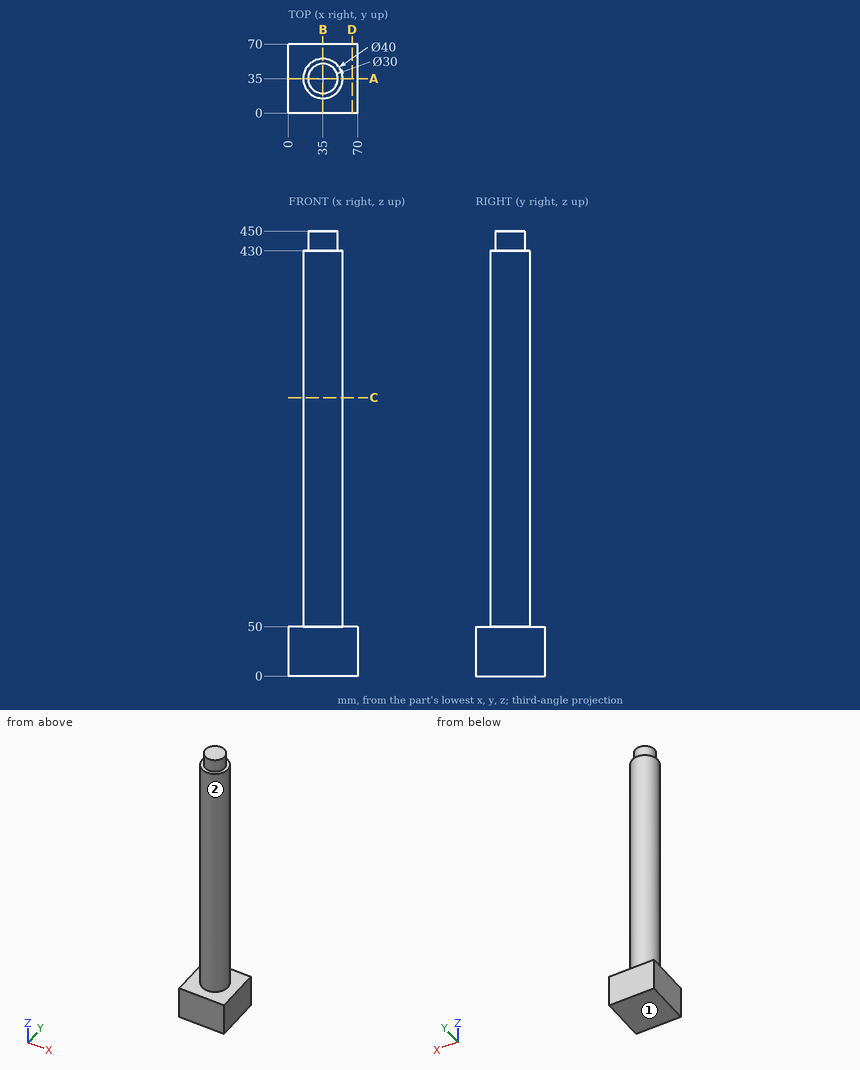
The figure shows three views and two pictorial views of one solid part (mm, origin at its lowest corner). Answer the questions. A direction names the side the tool comes from. Coordinates: 2 decimals unless noted, no trailing zeros. Write each loop counter-clockwise with the first axis right and the second up, starting at its lowest first coordinate (ties: lowest second). Pieces come first, ordered by that corner, then holes. Notation, with made-up numbers: (9, 13.25) -> (33, 13.25) arc R29 ccw to (33, 51.25) -> close; hole circle Ø5 at (-7, -14). An arc over 180 degrees is marked (long way). Answer as a JSON object with one key per item and string values.
Q1. Consider line 1 (Z direction, x = 47, y = 15); line 2 (Z direction, x = 47.5, y = 45); line 3 (Y direction, x = 47, z = 386.5). Determine where each line is inside the solid, lowest interval first. Write a range as [from, to].
The answers:
{"line 1": "z = [0, 50]", "line 2": "z = [0, 430]", "line 3": "y = [19, 51]"}
Q2. The part is cut by section C-C on z = 281.5. Give the vertices of the cut face in (x, y).
The answers:
{"outline": "circle Ø40 at (35, 35)"}
Q3. Flat-ended cylindrical pins translate along their axes: pin 1 Ø2 at (y, z) = (21, 121.5) entering from +X; pin 2 Ø2 at (x, z) = (36.5, 273.5) entering from +Y; pin 3 Ø3 at (x, y) = (54.5, 8.5) entering from +Z. Find the tip coordinate at first contact, or state that the pin passes through.
The answers:
{"pin 1": "stops at x = 50.2", "pin 2": "stops at y = 54.99", "pin 3": "stops at z = 50"}
Q4. The part is cut by section D-D on x = 64.5. Give the vertices of the cut face in (y, z).
The answers:
{"outline": "(0, 0) -> (70, 0) -> (70, 50) -> (0, 50) -> close"}
Q5. The part is cut by section A-A on y = 35. Give the vertices of the cut face in (x, z).
The answers:
{"outline": "(0, 0) -> (70, 0) -> (70, 50) -> (55, 50) -> (55, 430) -> (50, 430) -> (50, 450) -> (20, 450) -> (20, 430) -> (15, 430) -> (15, 50) -> (0, 50) -> close"}
Q6. A tool of negligible diameter and unlimited length cuts with its end or side. For the marked faces 1 and 2, from which of +Z, -Z, +X, -X, +Y, -Y can it reach the whole face along a straight path? Write none if from no direction.
The answers:
{"face 1": "-Z, +X, -X, +Y, -Y", "face 2": "+Z"}
